The model under review builds one solid part; all positions refer to its coordinate system, in mm. A direction names the side the tool comes from. Give positions to 0.01 mm unless a question says otherwise; leave off trailing zeros. Order: outer loops, then holes, each group sorted by start corner. A loop starts at its lowest first (then second) coordinate and runs counter-clockwise, first axis right, second up.
```python
from build123d import *

# Parameters (mm, degrees)
SKIZZE1_R                         = 3.5
SKIZZE1_R_2                       = 2
AUFSATZ_LINEAR_AUSTRAGEN1_DEPTH   = 2.5
AUFSATZ_LINEAR_AUSTRAGEN1_2_DEPTH = 2.5
AUFSATZ_LINEAR_AUSTRAGEN1_3_DEPTH = 2.5
AUFSATZ_LINEAR_AUSTRAGEN1_4_DEPTH = 2.5
SKIZZE2_R                         = 5.5
SKIZZE2_R_2                       = 2
AUFSATZ_LINEAR_AUSTRAGEN3_DEPTH   = 1
SKIZZE3_R                         = 5.5
SKIZZE3_R_2                       = 3.5
AUFSATZ_LINEAR_AUSTRAGEN4_DEPTH   = 2.5
SKIZZE4_R                         = 3.5
SKIZZE4_R_2                       = 1.25
AUFSATZ_LINEAR_AUSTRAGEN7_DEPTH   = 1
SCHNITT_LINEAR_AUSTRAGEN1_DEPTH   = 1
AUFSATZ_LINEAR_AUSTRAGEN8_DEPTH   = 2


with BuildPart() as part:
    # Skizze1 → Aufsatz-Linear austragen1 (new body)
    with BuildSketch(Plane.XY):
        with Locations((0, 34)):
            Circle(SKIZZE1_R)
        with Locations((0, 34)):
            Circle(SKIZZE1_R_2, mode=Mode.SUBTRACT)
    extrude(amount=AUFSATZ_LINEAR_AUSTRAGEN1_DEPTH)



with BuildPart() as body_2:
    # Skizze1 → Aufsatz-Linear austragen1 2 (new body)
    with BuildSketch(Plane.XY):
        with Locations((68, 34)):
            Circle(SKIZZE1_R)
        with Locations((68, 34)):
            Circle(SKIZZE1_R_2, mode=Mode.SUBTRACT)
    extrude(amount=AUFSATZ_LINEAR_AUSTRAGEN1_2_DEPTH)


with BuildPart() as body_3:
    # Skizze1 → Aufsatz-Linear austragen1 3 (new body)
    with BuildSketch(Plane.XY):
        with Locations((68, 0)):
            Circle(SKIZZE1_R)
        with Locations((68, 0)):
            Circle(SKIZZE1_R_2, mode=Mode.SUBTRACT)
    extrude(amount=AUFSATZ_LINEAR_AUSTRAGEN1_3_DEPTH)


with BuildPart() as body_4:
    # Skizze1 → Aufsatz-Linear austragen1 4 (new body)
    with BuildSketch(Plane.XY):
        Circle(SKIZZE1_R)
        Circle(SKIZZE1_R_2, mode=Mode.SUBTRACT)
    extrude(amount=AUFSATZ_LINEAR_AUSTRAGEN1_4_DEPTH)


with BuildPart() as part_1:
    add(part.part)

    add(body_2.part)  # Aufsatz-Linear austragen3 merges body 2

    add(body_3.part)  # Aufsatz-Linear austragen3 merges body 3

    add(body_4.part)  # Aufsatz-Linear austragen3 merges body 4
    # Skizze2 → Aufsatz-Linear austragen3 (add)
    # profile 1 of 4: a face of its own
    with BuildSketch(Plane.XY.offset(2.5)):
        with Locations((0, 34)):
            Circle(SKIZZE2_R)
        with Locations((0, 34)):
            Circle(SKIZZE2_R_2, mode=Mode.SUBTRACT)
    # profile 2 of 4: a face of its own
    with BuildSketch(Plane.XY.offset(2.5)):
        with Locations((68, 34)):
            Circle(SKIZZE2_R)
        with Locations((68, 34)):
            Circle(SKIZZE2_R_2, mode=Mode.SUBTRACT)
    # profile 3 of 4: a face of its own
    with BuildSketch(Plane.XY.offset(2.5)):
        with Locations((68, 0)):
            Circle(SKIZZE2_R)
        with Locations((68, 0)):
            Circle(SKIZZE2_R_2, mode=Mode.SUBTRACT)
    # profile 4 of 4: a face of its own
    with BuildSketch(Plane.XY.offset(2.5)):
        Circle(SKIZZE2_R)
        Circle(SKIZZE2_R_2, mode=Mode.SUBTRACT)
    extrude(amount=AUFSATZ_LINEAR_AUSTRAGEN3_DEPTH)

    # Skizze3 → Aufsatz-Linear austragen4 (add)
    # profile 1 of 4: a face of its own
    with BuildSketch(Plane.XY.offset(3.5)):
        with Locations((0, 34)):
            Circle(SKIZZE3_R)
        with Locations((0, 34)):
            Circle(SKIZZE3_R_2, mode=Mode.SUBTRACT)
    # profile 2 of 4: a face of its own
    with BuildSketch(Plane.XY.offset(3.5)):
        with Locations((68, 34)):
            Circle(SKIZZE3_R)
        with Locations((68, 34)):
            Circle(SKIZZE3_R_2, mode=Mode.SUBTRACT)
    # profile 3 of 4: a face of its own
    with BuildSketch(Plane.XY.offset(3.5)):
        with Locations((68, 0)):
            Circle(SKIZZE3_R)
        with Locations((68, 0)):
            Circle(SKIZZE3_R_2, mode=Mode.SUBTRACT)
    # profile 4 of 4: a face of its own
    with BuildSketch(Plane.XY.offset(3.5)):
        Circle(SKIZZE3_R)
        Circle(SKIZZE3_R_2, mode=Mode.SUBTRACT)
    extrude(amount=AUFSATZ_LINEAR_AUSTRAGEN4_DEPTH)

    # Skizze4 → Aufsatz-Linear austragen7 (add)
    with BuildSketch(Plane.XY.offset(6)):
        with BuildLine():
            Line((-4.5, 45), (74.5, 45))
            ThreePointArc((74.5, 45), (76.621320344, 44.121320344), (77.5, 42))
            Line((77.5, 42), (77.5, -8))
            ThreePointArc((77.5, -8), (76.621320344, -10.121320344), (74.5, -11))
            Line((74.5, -11), (-4.5, -11))
            ThreePointArc((-4.5, -11), (-6.621320344, -10.121320344), (-7.5, -8))
            Line((-7.5, -8), (-7.5, 42))
            ThreePointArc((-7.5, 42), (-6.621320344, 44.121320344), (-4.5, 45))
        make_face()
        with Locations((0, 34)):
            Circle(SKIZZE4_R, mode=Mode.SUBTRACT)
        with Locations((68, 34)):
            Circle(SKIZZE4_R, mode=Mode.SUBTRACT)
        with Locations((68, 0)):
            Circle(SKIZZE4_R, mode=Mode.SUBTRACT)
        with Locations((74.5, 42)):
            Circle(SKIZZE4_R_2, mode=Mode.SUBTRACT)
        with Locations((74.5, -8)):
            Circle(SKIZZE4_R_2, mode=Mode.SUBTRACT)
        with Locations((16.5, 42)):
            Circle(SKIZZE4_R_2, mode=Mode.SUBTRACT)
        with Locations((16.5, -8)):
            Circle(SKIZZE4_R_2, mode=Mode.SUBTRACT)
        Circle(SKIZZE4_R, mode=Mode.SUBTRACT)
        with BuildLine():
            Line((5.5, 0), (62.5, 0))
            ThreePointArc((62.5, 0), (64.110912703, 3.889087297), (68, 5.5))
            Line((68, 5.5), (68, 28.5))
            ThreePointArc((68, 28.5), (64.110912703, 30.110912703), (62.5, 34))
            Line((62.5, 34), (5.5, 34))
            ThreePointArc((5.5, 34), (3.889087297, 30.110912703), (0, 28.5))
            Line((0, 28.5), (0, 5.5))
            ThreePointArc((0, 5.5), (3.889087297, 3.889087297), (5.5, 0))
        make_face(mode=Mode.SUBTRACT)
    extrude(amount=AUFSATZ_LINEAR_AUSTRAGEN7_DEPTH)

    # Skizze6 → Schnitt-Linear austragen1 (cut)
    with BuildSketch(Plane.XY.offset(7)):
        with BuildLine():
            Line((16.889911487, 44.974553585), (51.565115858, 40.429246163))
            ThreePointArc((51.565115858, 40.429246163), (61.389636667, 40.61691637), (70.723351618, 43.689080824))
            Line((70.723351618, 43.689080824), (72.267833458, 44.468613251))
            ThreePointArc((72.267833458, 44.468613251), (73.352727218, 44.865322658), (74.5, 45))
            Line((74.5, 45), (74.5, 49.663390108))
            Line((74.5, 49.663390108), (16.5, 49.663390108))
            Line((16.5, 49.663390108), (16.5, 45))
            ThreePointArc((16.5, 45), (16.695370473, 44.993631637), (16.889911487, 44.974553585))
        make_face()
        with BuildLine():
            Line((74.5, -11), (74.5, -15.663390108))
            Line((74.5, -15.663390108), (16.5, -15.663390108))
            Line((16.5, -15.663390108), (16.5, -11))
            ThreePointArc((16.5, -11), (16.695370473, -10.993631637), (16.889911487, -10.974553585))
            Line((16.889911487, -10.974553585), (51.565115858, -6.429246163))
            ThreePointArc((51.565115858, -6.429246163), (61.389636667, -6.61691637), (70.723351618, -9.689080824))
            Line((70.723351618, -9.689080824), (72.267833458, -10.468613251))
            ThreePointArc((72.267833458, -10.468613251), (73.352727218, -10.865322658), (74.5, -11))
        make_face()
    extrude(amount=-SCHNITT_LINEAR_AUSTRAGEN1_DEPTH, mode=Mode.SUBTRACT)

    # Skizze7 → Aufsatz-Linear austragen8 (add)
    with BuildSketch(Plane(origin=(0, 0, 6), x_dir=(-1, 0, 0), z_dir=(0, 0, -1))):
        with BuildLine():
            Line((-77.5, 42), (-77.5, -8))
            ThreePointArc((-77.5, -8), (-76.621320344, -10.121320344), (-74.5, -11))
            Line((-74.5, -11), (-75.5, -11))
            ThreePointArc((-75.5, -11), (-77.621320344, -10.121320344), (-78.5, -8))
            Line((-78.5, -8), (-78.5, 42))
            ThreePointArc((-78.5, 42), (-77.621320344, 44.121320344), (-75.5, 45))
            Line((-75.5, 45), (-74.5, 45))
            ThreePointArc((-74.5, 45), (-76.621320344, 44.121320344), (-77.5, 42))
        make_face()
        with BuildLine():
            Line((4.5, -11), (-16.5, -11))
            Line((-16.5, -11), (-11.006587527, -11.72008944))
            ThreePointArc((-11.006587527, -11.72008944), (-8.866636381, -11.929948007), (-6.717561173, -12))
            Line((-6.717561173, -12), (4.5, -12))
            ThreePointArc((4.5, -12), (7, -10.75), (7.5, -8))
            ThreePointArc((7.5, -8), (6.621320344, -10.121320344), (4.5, -11))
        make_face()
        with BuildLine():
            Line((-6.717561173, 46), (4.5, 46))
            ThreePointArc((4.5, 46), (7, 44.75), (7.5, 42))
            ThreePointArc((7.5, 42), (6.621320344, 44.121320344), (4.5, 45))
            Line((4.5, 45), (-16.5, 45))
            Line((-16.5, 45), (-11.006587527, 45.72008944))
            ThreePointArc((-11.006587527, 45.72008944), (-8.866636381, 45.929948007), (-6.717561173, 46))
        make_face()
    extrude(amount=-AUFSATZ_LINEAR_AUSTRAGEN8_DEPTH)


solid = part_1.part
```
Item 1: Clearance check with flat-ended pins moving along their axes: pin 1 Ø2 at (x, y) = (16.5, 42) entering from -Z; pin 2 Ø5.5 at (x, y) = (66.5, 32.5) entering from +Z; pin 3 Ø4 at (x, z) = (17, 4.5) entering from -Y; pin 4 Ø1 at (y, z) = (13, 6.5) entering from -X. State where each tip first meets the part, or that it passes through.
Values found:
pin 1: passes through
pin 2: stops at z = 7
pin 3: stops at y = -11.11
pin 4: stops at x = -7.5
Item 2: Take a section at B-B (y = 10). Give the boundary of the cut face in (x, z).
Values found:
outline: (-7.5, 6) - (0, 6) - (0, 7) - (-7.5, 7) - close; (68, 6) - (78.5, 6) - (78.5, 8) - (77.5, 8) - (77.5, 7) - (68, 7) - close
Item 3: For faces 1 (the flat face through (36, 37, 6)), 2 (the flat face through (2, -2, 3.5)), 3 (the flat face through (33.985, 42.734, 6.507)), 4 (the cylindrical face through (16.23, -9.22, 6.49)), list the 3-axis set-ups (+Z, -Z, +X, -X, +Y, -Y) from which the entire face can be reached by the end or side of a thin tool; tool diameter is ignored.
Values found:
face 1: -Z
face 2: +Z
face 3: +Z, -Z, +Y
face 4: +Z, -Z
Item 4: Take a section at A-A (z = 1). Give the boundary of the cut face in (x, y), and give its area (3 significant figures).
Values found:
outline: circle Ø7 at (0, 0); circle Ø7 at (0, 34); circle Ø7 at (68, 0); circle Ø7 at (68, 34); hole circle Ø4 at (0, 0); hole circle Ø4 at (0, 34); hole circle Ø4 at (68, 0); hole circle Ø4 at (68, 34)
area: 104 mm2
Item 5: Take a section at C-C (z = 5). Give the boundary of the cut face in (x, y).
Values found:
outline: circle Ø11 at (0, 0); circle Ø11 at (0, 34); circle Ø11 at (68, 0); circle Ø11 at (68, 34); hole circle Ø7 at (0, 0); hole circle Ø7 at (0, 34); hole circle Ø7 at (68, 0); hole circle Ø7 at (68, 34)
Item 6: Draft analysis for pull direction X (two halves, no side actions). For faces 5 (the cylindrical face through (65.42, 36.365, 5.226)), 6 (the cylindrical face through (77.64, 44.1, 6.99)), 7 (the flat face through (2, 32, 0)), state which applies: released by +X, released by -X, zero draft, split by the parting line, or undercut.
Values found:
face 5: undercut
face 6: released by +X
face 7: zero draft
Item 7: Take a section at D-D (x = 38). Give the boundary of the cut face in (y, z), and give its area (3 significant figures).
Values found:
outline: (-8.21, 6) - (0, 6) - (0, 7) - (-8.21, 7) - close; (34, 6) - (42.21, 6) - (42.21, 7) - (34, 7) - close
area: 16.4 mm2
Item 8: For line 1 (Y direction, x = 0, z = 0.8); line 2 (Y direction, x = 16.5, z = 6.45); line 3 (X direction, y = 35, z = 2), list the stretches that pass through material, from the lowest coordinate up.
Values found:
line 1: y = -3.5 to -2, 2 to 3.5, 30.5 to 32, 36 to 37.5
line 2: y = -11 to -9.25, -6.75 to 0, 34 to 40.75, 43.25 to 45
line 3: x = -3.35 to -1.73, 1.73 to 3.35, 64.65 to 66.27, 69.73 to 71.35
